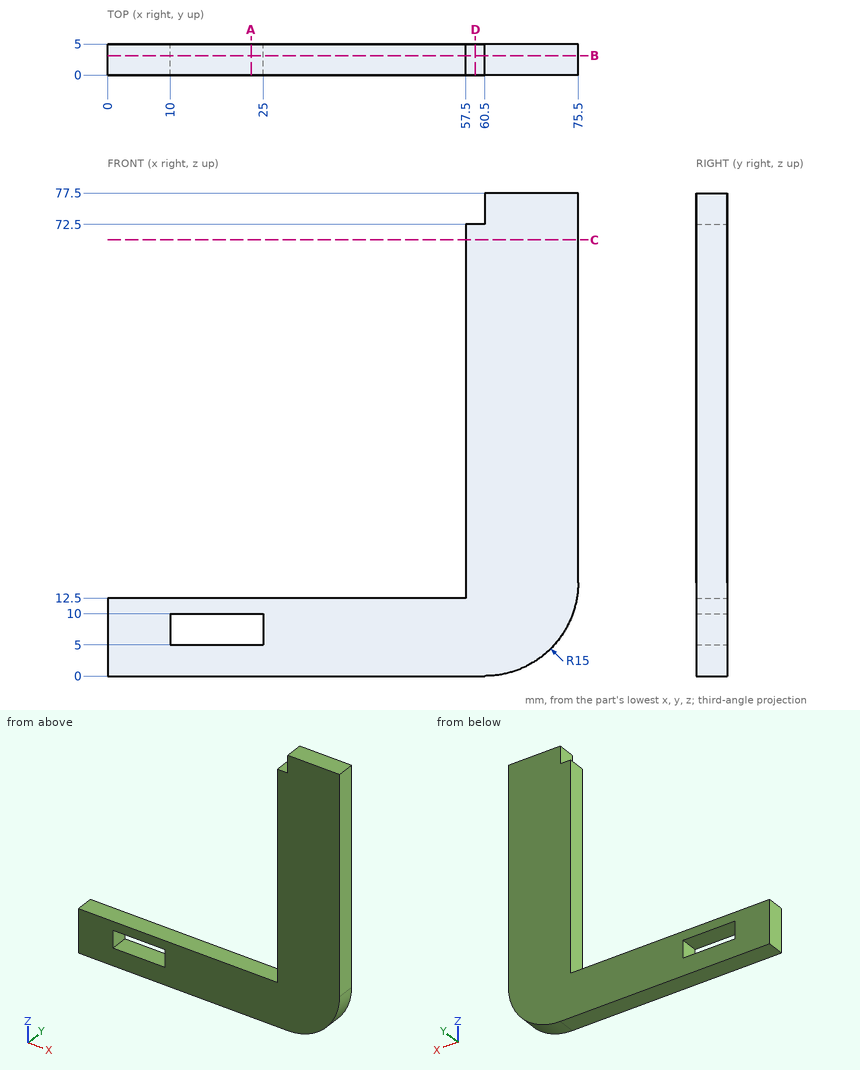
Geometry check sheet. Reference: drawing and pictorial views, mm from the part's lowest x, y, z. Round coordinates to 2 decimals unless told otherwise and drop trailing zeros. Loops run counter-clockwise (first coordinate to the right, second up) from the corner with the lowest first, then second, coordinate; pieces in that order, holes last. Notation, with made-up numbers: (71, 84) - (96, 84) arc R21 cw to (96, 111) - close; hole circle Ø3 at (45, 56.5). An arc over 180 degrees is marked (long way). Use a Markdown table: item, result.
Q1. Material ranges on line 1 (Z direction, x = 20.5, y = 1.4); line 2 (X direction, y = 3.1, z = 62); line 3 (Z direction, x = 55.5, y = 4.35), recorded low to high.
Solutions:
| item | result |
|---|---|
| line 1 | z = 0 to 5, 10 to 12.5 |
| line 2 | x = 57.5 to 75.5 |
| line 3 | z = 0 to 12.5 |
Q2. Go/stop test with flat-tipped pins: P1, Ø1.5, axis at y = 3.5, z = 6.5, coming from the +X side; P2, Ø6, axis at x = 61.5, z = 15, coming from the -Y side; P3, Ø1.5, axis at y = 2, z = 53.5, coming from the -X side; P4, Ø1.5, axis at x = 15.5, y = 3.5, coming from the +Z side. Record where each tip stops, or that it passes through.
Solutions:
| item | result |
|---|---|
| P1 | stops at x = 73.34 |
| P2 | stops at y = 0 |
| P3 | stops at x = 57.5 |
| P4 | stops at z = 12.5 |
Q3. Cross-section at B-B on y = 3.15. Record the cut outline in (x, z), plus the area to 3 significant figures.
Solutions:
| item | result |
|---|---|
| outline | (0, 0) - (60.5, 0) arc R15 ccw to (75.5, 15) - (75.5, 77.5) - (60.5, 77.5) - (60.5, 72.5) - (57.5, 72.5) - (57.5, 12.5) - (0, 12.5) - close; hole (10, 5) - (25, 5) - (25, 10) - (10, 10) - close |
| area | 1,980 mm2 |
Q4. Cross-section at C-C on z = 70. Record the cut outline in (x, y).
Solutions:
| item | result |
|---|---|
| outline | (57.5, 0) - (75.5, 0) - (75.5, 5) - (57.5, 5) - close |
Q5. Cross-section at A-A on x = 23. Record the cut outline in (y, z).
Solutions:
| item | result |
|---|---|
| outline | (0, 0) - (5, 0) - (5, 5) - (0, 5) - close; (0, 10) - (5, 10) - (5, 12.5) - (0, 12.5) - close |
Q6. Cross-section at D-D on x = 59. Record the cut outline in (y, z), plus the area to 4 significant figures.
Solutions:
| item | result |
|---|---|
| outline | (0, 0) - (5, 0) - (5, 72.5) - (0, 72.5) - close |
| area | 362.5 mm2 |
